Can you work these out from the model? Positions are in its coordinate system, mm. Give positions to 0.01 mm unless a question says otherwise; leave off trailing zeros. One line per question, with ' | ' between items.
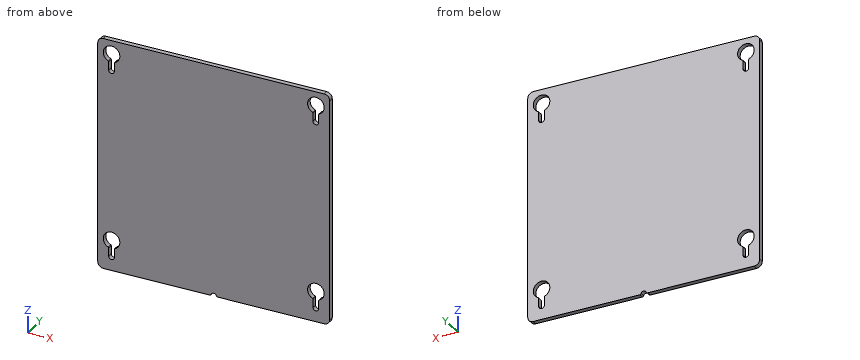
```python
from build123d import *

# Parameters (mm, degrees)
SKETCH1_W           = 266.7
SKETCH1_H           = 266.7
SKETCH1_R           = 3.2639
BOSS_EXTRUDE1_DEPTH = 5.588
FILLET1_R           = 6.35
CUT_EXTRUDE2_DEPTH  = 378.212149518
SKETCH6_R           = 3.302
CUT_EXTRUDE3_DEPTH  = 378.212149518
FILLET2_R           = 1.5875
FILLET3_R           = 0.762


with BuildPart() as part:
    # Sketch1 → Boss-Extrude1 (new body)
    with BuildSketch(Plane(origin=(0, 0, 0), x_dir=(1, 0, 0), z_dir=(0, 1, 0))):
        with Locations((133.35, 133.35)):
            Rectangle(SKETCH1_W, SKETCH1_H)
        with Locations(Location((15.875, 250.825, 0), (0, 0, 270))):
            Circle(SKETCH1_R, mode=Mode.SUBTRACT)
        with Locations(Location((250.825, 250.825, 0), (0, 0, 270))):
            Circle(SKETCH1_R, mode=Mode.SUBTRACT)
        with Locations(Location((15.875, 15.875, 0), (0, 0, 270))):
            Circle(SKETCH1_R, mode=Mode.SUBTRACT)
        with Locations(Location((250.825, 15.875, 0), (0, 0, 270))):
            Circle(SKETCH1_R, mode=Mode.SUBTRACT)
    extrude(amount=BOSS_EXTRUDE1_DEPTH)

    # Fillet1
    fillet1_edges = [part.edges().sort_by_distance(p)[0] for p in [
        (0, 2.794, -266.7),
        (266.7, 2.794, -266.7),
        (266.7, 2.794, 0),
        (0, 2.794, 0),
    ]]
    fillet(fillet1_edges, radius=FILLET1_R)

    # Sketch5 → Cut-Extrude2 (cut, through all)
    with BuildSketch(Plane(origin=(0, 5.588, 0), x_dir=(1, 0, 0), z_dir=(0, 1, 0))):
        with BuildLine():
            Line((19.1389, 34.925), (19.1389, 24.823328436))
            ThreePointArc((19.1389, 24.823328436), (15.875, 6.35), (12.6111, 24.823328436))
            Line((12.6111, 24.823328436), (12.6111, 34.925))
            ThreePointArc((12.6111, 34.925), (15.875, 38.1889), (19.1389, 34.925))
        make_face()
        with BuildLine():
            Line((254.0889, 34.925), (254.0889, 24.823328436))
            ThreePointArc((254.0889, 24.823328436), (250.825, 6.35), (247.5611, 24.823328436))
            Line((247.5611, 24.823328436), (247.5611, 34.925))
            ThreePointArc((247.5611, 34.925), (250.825, 38.1889), (254.0889, 34.925))
        make_face()
        with BuildLine():
            Line((19.1389, 250.825), (19.1389, 240.723328436))
            ThreePointArc((19.1389, 240.723328436), (15.875, 222.25), (12.6111, 240.723328436))
            Line((12.6111, 240.723328436), (12.6111, 250.825))
            ThreePointArc((12.6111, 250.825), (15.875, 254.0889), (19.1389, 250.825))
        make_face()
        with BuildLine():
            Line((254.0889, 250.825), (254.0889, 240.723328436))
            ThreePointArc((254.0889, 240.723328436), (250.825, 222.25), (247.5611, 240.723328436))
            Line((247.5611, 240.723328436), (247.5611, 250.825))
            ThreePointArc((247.5611, 250.825), (250.825, 254.0889), (254.0889, 250.825))
        make_face()
    extrude(amount=-CUT_EXTRUDE2_DEPTH, mode=Mode.SUBTRACT)

    # Sketch6 → Cut-Extrude3 (cut, through all)
    with BuildSketch(Plane(origin=(0, 5.588, 0), x_dir=(1, 0, 0), z_dir=(0, 1, 0))):
        with Locations((133.35, 266.7)):
            Circle(SKETCH6_R)
    extrude(amount=-CUT_EXTRUDE3_DEPTH, mode=Mode.SUBTRACT)

    # Fillet2
    fillet2_edges = [part.edges().sort_by_distance(p)[0] for p in [
        (130.048, 2.794, -266.7),
        (136.652, 2.794, -266.7),
    ]]
    fillet(fillet2_edges, radius=FILLET2_R)

    # Fillet3
    fillet3_edges = [part.edges().sort_by_distance(p)[0] for p in [
        (254.0889, 2.794, -24.823328436),
        (247.5611, 2.794, -24.823328436),
        (19.1389, 2.794, -240.723328436),
        (12.6111, 2.794, -240.723328436),
        (254.0889, 2.794, -240.723328436),
        (247.5611, 2.794, -240.723328436),
        (19.1389, 2.794, -24.823328436),
        (12.6111, 2.794, -24.823328436),
    ]]
    fillet(fillet3_edges, radius=FILLET3_R)


solid = part.part
```
(1) If I drill on line 1 (X direction, y = 2.95, z = -34.5); line 2 (Z direction, x = 246.5, y = 3.9); line 3 (X direction, y = 2.6, z = -23.5), over which ranges is the centre line in solid material (lowest first)?
Answer below:
line 1: 0 to 12.61, 19.14 to 247.56, 254.09 to 266.7 | line 2: -266.7 to -240.26, -223.29 to -24.36, -7.39 to 0 | line 3: 0 to 10.17, 21.58 to 245.12, 256.53 to 266.7
(2) Will this pin go through, and if not, where does the flat tip stop? pin 1 (17 mm diameter, centred on x = 250.825, z = -231.775, fed in from +Y).
Answer below:
pin 1: through
(3) Imagine slicing it at A-A (y = 2.7). Count the separate pieces of the cut face and the enclosed holes in it, and give its area (3 significant figures).
Answer below:
separate pieces: 1 | enclosed holes: 4 | area: 69,600 mm^2
